Part model, mm, in its own coordinate system. A direction names the side the tool comes from. Give positions to 0.01 mm unless a question says otherwise; leave off trailing zeros. Write each loop counter-clockwise with the first axis right and the second up, starting at its lowest first coordinate (ties: lowest second). Pieces come first, ordered by that corner, then holes. Notation, with made-up numbers: M 17,56.25 L 65,56.25 A17 ccw 65,63.25 Z; hole C 66,58 d4. An arc over 180 degrees is marked long. Answer as CSV lines item,"result". Start each with the question number.
Item 1: Two-plate mould, pull along Y, no slides. Class faces 1 (the cylindrical face through (10.382, -19.961, 25.918)), 2 (the flat face through (0, 0, 0)), 3 (the cylindrical face through (23.846, 7.509, 24.664)): +Y half, -Y half, draft (parallel to the pull), parting line (faces both ways), or undercut.
Item 2: Wall check: L1, parallel to Y at x = 0, z = 29.5; L2, parallel to Z at x = -11, y = 13.5; L3, parallel to X at y = -20, z = 35. Give the ranges that are in metal, low to high. Write a range as from..to.
Item 3: Pin check, flat tips, straight feed: pin 1 (2 mm diameter, centred on y = -12, z = 19.5, fed in from +X); pin 2 (3 mm diameter, centred on y = 12, z = 25, fed in from +X); pin 3 (1.5 mm diameter, centred on y = -13, z = 10, fed in from +X); pin 4 (3 mm diameter, centred on x = 9.5, y = 10, fed in from -Z). Stop position of each tip, or through.
Item 4: Band-saw the part on B-B, the plane z = 37. List the corners of the cut face in (x, y).
Item 5: 3-axis set-ups, long thin cutter, end or side, ignore diameter. For faces 4 (the flat face through (0, 0, 2.5)), 5 (the flat face through (14, -18, 50)): which of +Z, -Z, +X, -X, +Y, -Y reach the whole face in a straight line?
Item 6: Band-saw the part on A-A, the plane x = 0. List the corners of the cut face in (y, z), then the cut area to 3 significant figures.
from build123d import *

# Parameters (mm, degrees)
F0_R     = 25
F1_DEPTH = 50
F2_T     = -2.5
F3_R     = 1


with BuildPart() as f1:
    # F0 (on Top) → F1 (new body)
    with BuildSketch(Plane.XY):
        Circle(F0_R)
    extrude(amount=F1_DEPTH)

    # F2
    f2_openings = [f1.faces().sort_by_distance(p)[0] for p in [
        (0, 0, 50),
    ]]
    offset(amount=F2_T, openings=f2_openings)

    # F3
    f3_edges = [f1.edges().sort_by_distance(p)[0] for p in [
        (25, 0, 25),
        (-25, 0, 0),
        (-25, 0, 50),
    ]]
    fillet(f3_edges, radius=F3_R)


solid = f1.part
Output:
1,face 1,"undercut"
1,face 2,"draft"
1,face 3,"parting line"
2,L1,"-25..-22.5, 22.5..25"
2,L2,"0..2.5"
2,L3,"-15..-10.31, 10.31..15"
3,pin 1,"x = 22.45"
3,pin 2,"x = 22.69"
3,pin 3,"x = 21.79"
3,pin 4,"z = 0"
4,outline,"C 0,0 d50; hole C 0,0 d45"
5,face 4,"+Z"
5,face 5,"+Z, +X, -X, +Y, -Y"
6,outline,"M -25,1 A1 ccw -24,0 L 24,0 A1 ccw 25,1 L 25,49 A1 ccw 24,50 L 22.5,50 L 22.5,2.5 L -22.5,2.5 L -22.5,50 L -24,50 A1 ccw -25,49 Z"
6,area,"362 mm²"
